```python
from build123d import *

# Parameters (mm, degrees)
SKETCH1_R               = 25.146
BOSS_EXTRUDE1_DEPTH     = 2.54
SKETCH2_R               = 23.622
BOSS_EXTRUDE2_DEPTH     = 2.54
SKETCH3_R               = 3.2512
SKETCH3_R_2             = 4.191
CUT_EXTRUDE1_DEPTH      = 1
CUT_EXTRUDE1_DEPTH_BACK = 6.08
SKETCH4_R               = 2.8575
CUT_EXTRUDE2_DEPTH      = 5.08
CHAMFER1_SIZE           = 0.508


with BuildPart() as part:
    # Sketch1 → Boss-Extrude1 (new body)
    with BuildSketch(Plane(origin=(0, 0, 0), x_dir=(1, 0, 0), z_dir=(0, 1, 0))):
        Circle(SKETCH1_R)
    extrude(amount=BOSS_EXTRUDE1_DEPTH)

    # Sketch2 → Boss-Extrude2 (add)
    with BuildSketch(Plane(origin=(0, 2.54, 0), x_dir=(1, 0, 0), z_dir=(0, 1, 0))):
        Circle(SKETCH2_R)
    extrude(amount=BOSS_EXTRUDE2_DEPTH)

    # Sketch3 → Cut-Extrude1 (cut, two sides)
    with BuildSketch(Plane.XZ) as cut_extrude1_sk:
        Circle(SKETCH3_R)
        with Locations((-12.537653487, 3.45997074)):
            Circle(SKETCH3_R_2)
    extrude(amount=CUT_EXTRUDE1_DEPTH, mode=Mode.SUBTRACT)
    extrude(cut_extrude1_sk.sketch, amount=-CUT_EXTRUDE1_DEPTH_BACK, mode=Mode.SUBTRACT)

    # Sketch4 → Cut-Extrude2 (cut)
    with BuildSketch(Plane.XZ):
        with Locations((-12.512560688, -15.196547307)):
            Circle(SKETCH4_R)
        with Locations((-15.019030103, 12.725091739)):
            Circle(SKETCH4_R)
    extrude(amount=-CUT_EXTRUDE2_DEPTH, mode=Mode.SUBTRACT)

    # Chamfer1
    chamfer1_edges = [part.edges().sort_by_distance(p)[0] for p in [
        (-25.146, 0, 0),
        (-23.622, 5.08, 0),
    ]]
    chamfer(chamfer1_edges, length=CHAMFER1_SIZE)


solid = part.part
```
Design review of the part built by this model. Coordinates are the model's own, in mm. Round coordinates to 2 decimals unless told otherwise and drop trailing zeros. Write each loop counter-clockwise with the first axis right and the second up, starting at its lowest first coordinate (ties: lowest second). Pieces come first, ordered by that corner, then holes.
Item 1: Clearance check with flat-ended pins moving along their axes: pin 1 Ø13.5 at (x, z) = (-12.54, 3.46) entering from +Y; pin 2 Ø2 at (y, z) = (1.5, 19) entering from -X. State where each tip first meets the part, or that it passes through.
Item 2: We need section B-B on z = 0. Write out the cut boundary in (x, y).
Item 3: For probe 1 along Z at (x, y) = (0, 1.6); probe 2 along X at (y, z) = (2.4, 3); probe 3 along X at (y, z) = (2.9, 1.5), list the stretches that pass through material, from the lowest coordinate up.
Item 4: We need section A-A on x = 0. Write out the cut boundary in (y, z), and give its area (3 significant figures).
Item 5: The part is to be moulded in two halves that separate along X. For faces 1 (the flat face through (19, 2.54, 15)), 2 (the cylindrical face through (-13.132, 2.504, -17.986)), 3 (the cylindrical face through (-13.7, 2.5, 10.19)), 4 (the cylindrical face through (-18.75, 3.54, 14.37)), say which applies: +X half, -X half, draft (parallel to the pull), parting line (faces both ways), or undercut.
Item 6: We need section C-C on y = 1.15. Write out the cut boundary in (x, z) (1 decimal), and give its area (3 significant figures).
Returned:
1. pin 1: stops at y = 5.08
1. pin 2: stops at x = -17.56
2. outline: (-25.15, 0.51) - (-24.64, 0) - (-14.9, 0) - (-14.9, 5.08) - (-23.11, 5.08) - (-23.62, 4.57) - (-23.62, 2.54) - (-25.15, 2.54) - close; (-10.17, 0) - (-3.25, 0) - (-3.25, 5.08) - (-10.17, 5.08) - close; (3.25, 0) - (24.64, 0) - (25.15, 0.51) - (25.15, 2.54) - (23.62, 2.54) - (23.62, 4.57) - (23.11, 5.08) - (3.25, 5.08) - close
3. probe 1: z = -25.15 to -3.25, 3.25 to 25.15
3. probe 2: x = -24.97 to -16.7, -8.37 to -1.25, 1.25 to 24.97
3. probe 3: x = -23.57 to -16.24, -8.83 to -2.88, 2.88 to 23.57
4. outline: (0, -24.64) - (0.51, -25.15) - (2.54, -25.15) - (2.54, -23.62) - (4.57, -23.62) - (5.08, -23.11) - (5.08, -3.25) - (0, -3.25) - close; (0, 3.25) - (5.08, 3.25) - (5.08, 23.11) - (4.57, 23.62) - (2.54, 23.62) - (2.54, 25.15) - (0.51, 25.15) - (0, 24.64) - close
4. area: 214 mm2
5. face 1: draft
5. face 2: undercut
5. face 3: undercut
5. face 4: parting line
6. outline: circle Ø50.3 at (0, 0); hole circle Ø5.7 at (-15, 12.7); hole circle Ø8.4 at (-12.5, 3.5); hole circle Ø5.7 at (-12.5, -15.2); hole circle Ø6.5 at (0, 0)
6. area: 1,850 mm2
